Geometry check sheet. Reference: the model listing, model coordinates, mm. A direction names the side the tool comes from. Round coordinates to 2 decimals unless told otherwise and drop trailing zeros. Order: outer loops, then holes, each group sorted by start corner. A loop starts at its lowest first (then second) coordinate and runs counter-clockwise, first axis right, second up. Notation, with made-up numbers: (-3.75, 4.5) - (13.25, 4.5) arc R10 cw to (13.25, 21.5) - close; hole circle Ø2 at (76, 38.5). An arc over 180 degrees is marked (long way). Write each question's results on one line, items separated by ' | '.
```python
from build123d import *

# Parameters (mm, degrees)
CROQUIS1_W              = 100
CROQUIS1_H              = 100
CROQUIS1_W_2            = 92
CROQUIS1_H_2            = 92
SALIENTE_EXTRUIR2_DEPTH = 1500
CORTAR_EXTRUIR2_DEPTH   = 180


with BuildPart() as part:
    # Croquis1 → Saliente-Extruir2 (new body)
    with BuildSketch(Plane.XY):
        with Locations((-19.634513149, 9.769055649)):
            Rectangle(CROQUIS1_W, CROQUIS1_H)
        with Locations((-19.634513149, 9.769055649)):
            Rectangle(CROQUIS1_W_2, CROQUIS1_H_2, mode=Mode.SUBTRACT)
    extrude(amount=SALIENTE_EXTRUIR2_DEPTH)

    # Croquis2 → Cortar-Extruir2 (cut)
    with BuildSketch(Plane.ZY.offset(69.634513149)):
        Polygon((1500, -40.230944351), (1400, 59.769055649), (1500, 59.769055649), align=None)
        Polygon((0, -40.230944351), (100, 59.769055649), (0, 59.769055649), align=None)
    extrude(amount=-CORTAR_EXTRUIR2_DEPTH, mode=Mode.SUBTRACT)


solid = part.part
```
(1) Access from +Z, -Z, +X, -X, +Y, -Y to the whole of each face (thin tool, end or side, straight path). Record for faces 5 (the face through (28.28, 5.83, 46.06)), 6 (the face through (26.365, 9, 740)).
Answers follow:
face 5: -Z, +X, -X, +Y | face 6: +Z, -Z
(2) Draft check along X on faces 1 (the face through (-20, 55.769, 741)), 2 (the face through (-69.635, 9, 740)), 3 (the face through (-20, -40.231, 740)), 4 (the face through (30.365, 9, 740)). Enter one of: released by +X, released by -X, zero draft, split by the parting line, or undercut.
Answers follow:
face 1: undercut | face 2: released by -X | face 3: zero draft | face 4: released by +X
(3) Section check A-A (x = -44.5). Record the cut outline in (y, z), then the cut area to 3 significant figures.
Answers follow:
outline: (-40.23, 0) - (-36.23, 4) - (-36.23, 1496) - (-40.23, 1500) - close; (55.77, 96) - (59.77, 100) - (59.77, 1400) - (55.77, 1404) - close | area: 11,200 mm²
(4) Section check C-C (z = 448). Record the cut outline in (x, y), then the cut area to 3 significant figures.
Answers follow:
outline: (-69.63, -40.23) - (30.37, -40.23) - (30.37, 59.77) - (-69.63, 59.77) - close; hole (-65.63, -36.23) - (26.37, -36.23) - (26.37, 55.77) - (-65.63, 55.77) - close | area: 1,540 mm²
(5) Section check B-B (y = 35). Record the cut outline in (x, z).
Answers follow:
outline: (-69.63, 75.23) - (-65.63, 75.23) - (-65.63, 1424.77) - (-69.63, 1424.77) - close; (26.37, 75.23) - (30.37, 75.23) - (30.37, 1424.77) - (26.37, 1424.77) - close
(6) Material ranges on line 1 (X direction, y = 12, z = 758); line 2 (Y direction, x = -5, z = 392); line 3 (Z direction, x = 26.5, y = 19), recorded low to high.
Answers follow:
line 1: -69.63 to -65.63, 26.37 to 30.37 | line 2: -40.23 to -36.23, 55.77 to 59.77 | line 3: 59.23 to 1440.77
